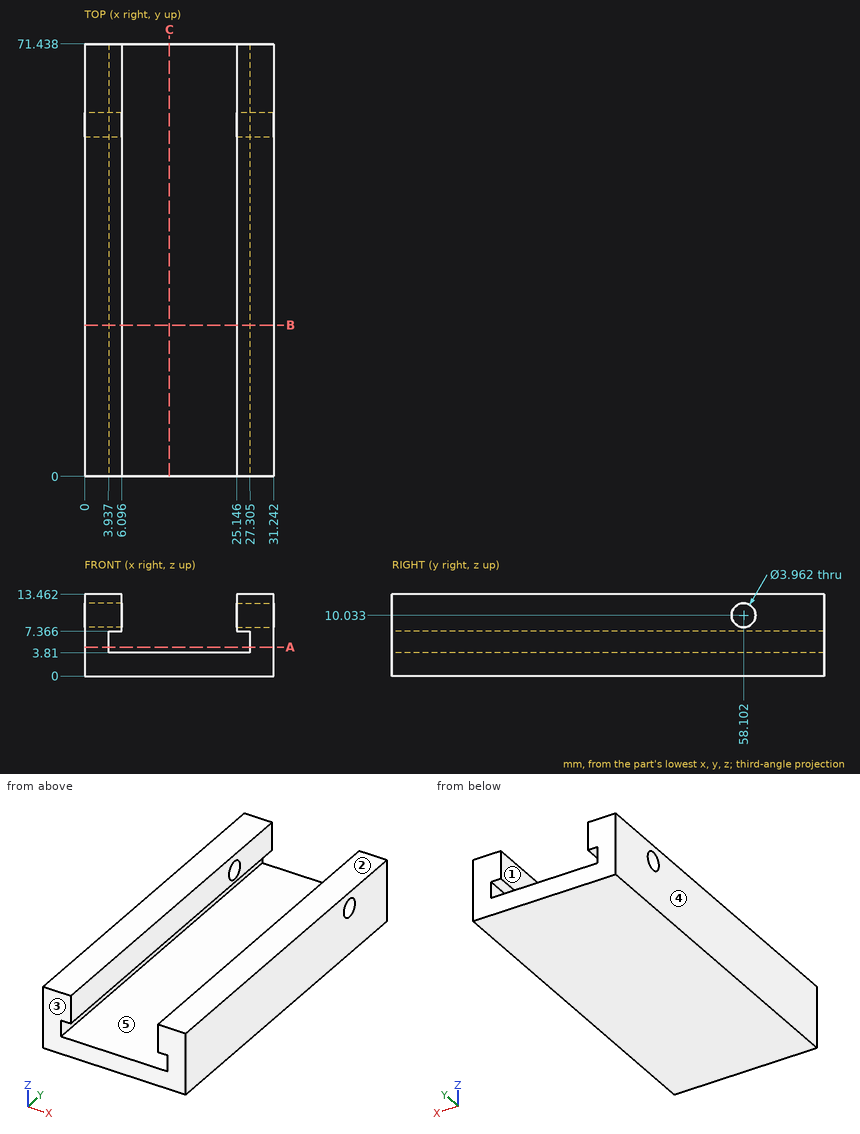
Answer from the drawing. Dimensions are ordinates in mm from the lowest x, y and z of the part. A direction names the side the tool comes from. Give positions to 0.01 mm unless a question says otherwise; leave off trailing zeros. Order: outer loops, then holes, each group sorted by start corner. A loop starts at its lowest first (then second) coordinate and runs counter-clockwise, first axis right, second up. Notation, with made-up numbers: (-11.75, 88.25) - (14.25, 88.25) arc R26 cw to (14.25, 125.25) - close; hole circle Ø11 at (-37.75, 79). An arc over 180 degrees is marked (long way). One line per item, written item: value. Start each with the question number.
1. Which of the six approach directions +Z, -Z, +X, -X, +Y, -Y give full straight-line access (tool end or side, diameter ignored) to the marked faces 1 and 2?
2. Consider line 1 (X direction, y = 15, z = 4.25) (1 decimal); line 2 (X direction, y = 52.5, z = 11.5) (1 decimal); line 3 (Z direction, x = 26, y = 35.5) (1 decimal). Determine where each line is inside the solid, lowest interval first.
3. For a pull along X with two mould halves and no side action, classify the marked faces 3, 4 and 5 as released by +X, released by -X, zero draft, split by the parting line, or undercut.
4. Section C-C, the plane x = 14 is taken. Write down the section's boundary in (y, z).
5. Section A-A, the plane z = 4.75 is taken. Write down the section's boundary in (x, y) (1 decimal).
6. Section B-B, the plane y = 25 is taken. Write down the section's boundary in (x, z) (1 decimal), then the cut area to 3 significant figures.
7. Each of these flat-tipped pins is pushed along its axis until it touches: pin 1 Ø2 at (x, y) = (11, 61.5) entering from +Z; pin 2 Ø2 at (x, z) = (22, 5) entering from +Y. Where does it stop, or does it pass through?
Filled sheet:
1. face 1: +Z, +Y, -Y
1. face 2: +Z, +X, -X, +Y, -Y
2. line 1: 0 to 3.9, 27.3 to 31.2
2. line 2: 0 to 6.1, 25.1 to 31.2
2. line 3: 0 to 3.8, 7.4 to 13.5
3. face 3: zero draft
3. face 4: released by -X
3. face 5: undercut
4. outline: (0, 0) - (71.44, 0) - (71.44, 3.81) - (0, 3.81) - close
5. outline: (0, 0) - (3.9, 0) - (3.9, 71.4) - (0, 71.4) - close; (27.3, 0) - (31.2, 0) - (31.2, 71.4) - (27.3, 71.4) - close
6. outline: (0, 0) - (31.2, 0) - (31.2, 13.5) - (25.1, 13.5) - (25.1, 7.4) - (27.3, 7.4) - (27.3, 3.8) - (3.9, 3.8) - (3.9, 7.4) - (6.1, 7.4) - (6.1, 13.5) - (0, 13.5) - close
6. area: 221 mm²
7. pin 1: z = 3.81
7. pin 2: through
